Drawing for the job (mm, zero at the part's lowest x, y, z). Round coordinates to 2 decimals unless told otherwise and drop trailing zeros. Loops run counter-clockwise (first coordinate to the right, second up) from the corner with the lowest first, then second, coordinate; pieces in that order, holes last. Notation, with made-up numbers: M 12.25,2.5 L 30.25,2.5 A20 ccw 30.25,30.5 Z; hole C 47,89.25 d11. An arc over 180 degrees is marked long. Write each question's results on one line, items separated by ' | '.
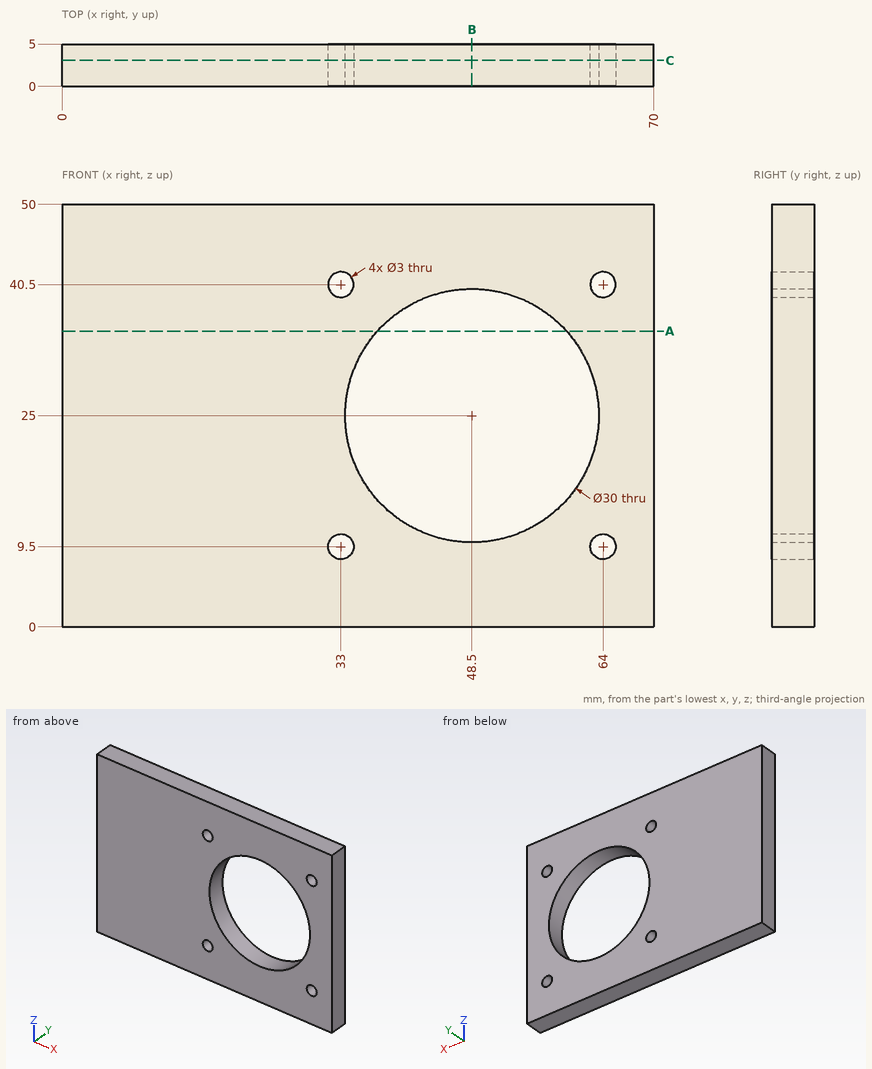
Item 1: Band-saw the part on A-A on z = 35. Give the cut face in (x, y).
Filled sheet:
outline: M 0,0 L 37.32,0 L 37.32,5 L 0,5 Z; M 59.68,0 L 70,0 L 70,5 L 59.68,5 Z
Item 2: Band-saw the part on C-C on y = 3.05. Give the cut face in (x, z).
Filled sheet:
outline: M 0,0 L 70,0 L 70,50 L 0,50 Z; hole C 33,9.5 d3; hole C 33,40.5 d3; hole C 48.5,25 d30; hole C 64,9.5 d3; hole C 64,40.5 d3
Item 3: Wall check: L1, parallel to Z at x = 33, y = 2.05; L2, parallel to Z at x = 32.5, y = 4.6; L3, parallel to Z at x = 48.5, y = 3.75. Give the ranges that are in metal, low to high.
Filled sheet:
L1: 0 to 8, 11 to 39, 42 to 50 | L2: 0 to 8.09, 10.91 to 39.09, 41.91 to 50 | L3: 0 to 10, 40 to 50
Item 4: Band-saw the part on B-B on x = 48.5. Give the cut face in (y, z), and give its area (3 significant figures).
Filled sheet:
outline: M 0,0 L 5,0 L 5,10 L 0,10 Z; M 0,40 L 5,40 L 5,50 L 0,50 Z | area: 100 mm^2
Item 5: Drop a flat-ended pin along its axis: P1, Ø2.5, axis at x = 64, z = 40.5, coming from the -Y side. Give the stop position or say it passes through.
Filled sheet:
P1: through
